Verification items for the finished model (mm, model axes). A direction names the side the tool comes from. Round coordinates to 2 decimals unless told otherwise and drop trailing zeros. Write each loop counter-clockwise with the first axis right and the second up, starting at its lowest first coordinate (ties: lowest second). Pieces come first, ordered by that corner, then holes.
from build123d import *

# Parameters (mm, degrees)
SKETCH_W        = 200
SKETCH_H        = 90
SKETCH_W_2      = 60
SKETCH_H_2      = 67
PAD_DEPTH       = 5
SKETCH001_W     = 200
SKETCH001_H     = 90
SKETCH001_W_2   = 124
SKETCH001_H_2   = 67
PAD001_DEPTH    = 5
SKETCH002_W     = 41
SKETCH002_H     = 9.5
POCKET_DEPTH    = 10.001
SKETCH003_R     = 1.5625
POCKET001_DEPTH = 10.001
FILLET_R        = 30
FILLET001_R     = 3
FILLET002_R     = 3
POCKET002_DEPTH = 2
FILLET003_R     = 1
FILLET004_R     = 1


with BuildPart() as part:
    # Sketch → Pad (new body)
    with BuildSketch(Plane.XY):
        with Locations((100, -45)):
            Rectangle(SKETCH_W, SKETCH_H)
        with Locations((70, -38.5)):
            Rectangle(SKETCH_W_2, SKETCH_H_2, mode=Mode.SUBTRACT)
        with BuildLine():
            ThreePointArc((158.0113, -7.9887), (155.0113, -4.9887), (152.0113, -7.9887))
            Line((152.0113, -7.9887), (152.0113, -17.9887))
            ThreePointArc((152.0113, -17.9887), (155.0113, -20.9887), (158.0113, -17.9887))
            Line((158.0113, -7.9887), (158.0113, -17.9887))
        make_face(mode=Mode.SUBTRACT)
        with BuildLine():
            ThreePointArc((151, -31.5), (131.5, -12), (112, -31.5))
            Line((112, -31.5), (112, -41.5))
            ThreePointArc((112, -41.5), (131.5, -61), (151, -41.5))
            Line((151, -31.5), (151, -41.5))
        make_face(mode=Mode.SUBTRACT)
        with BuildLine():
            ThreePointArc((158.0113, -55.0113), (155.0113, -52.0113), (152.0113, -55.0113))
            Line((152.0113, -55.0113), (152.0113, -65.0113))
            ThreePointArc((152.0113, -65.0113), (155.0113, -68.0113), (158.0113, -65.0113))
            Line((158.0113, -55.0113), (158.0113, -65.0113))
        make_face(mode=Mode.SUBTRACT)
        with BuildLine():
            ThreePointArc((110.9887, -55.0113), (107.9887, -52.0113), (104.9887, -55.0113))
            Line((104.9887, -55.0113), (104.9887, -65.0113))
            ThreePointArc((104.9887, -65.0113), (107.9887, -68.0113), (110.9887, -65.0113))
            Line((110.9887, -55.0113), (110.9887, -65.0113))
        make_face(mode=Mode.SUBTRACT)
        with BuildLine():
            ThreePointArc((110.9887, -7.9887), (107.9887, -4.9887), (104.9887, -7.9887))
            Line((104.9887, -7.9887), (104.9887, -17.9887))
            ThreePointArc((104.9887, -17.9887), (107.9887, -20.9887), (110.9887, -17.9887))
            Line((110.9887, -7.9887), (110.9887, -17.9887))
        make_face(mode=Mode.SUBTRACT)
    extrude(amount=PAD_DEPTH)

    # Sketch001 → Pad001 (join)
    with BuildSketch(Plane(origin=(0, 0, 0), x_dir=(1, 0, 0), z_dir=(0, 0, -1))):
        with Locations((100, 45)):
            Rectangle(SKETCH001_W, SKETCH001_H)
        with Locations((102, 38.5)):
            Rectangle(SKETCH001_W_2, SKETCH001_H_2, mode=Mode.SUBTRACT)
    extrude(amount=PAD001_DEPTH)

    # Sketch002 → Pocket (cut, through all)
    with BuildSketch(Plane.XY.offset(5)):
        with Locations((70, -76.75)):
            Rectangle(SKETCH002_W, SKETCH002_H)
    extrude(amount=-POCKET_DEPTH, mode=Mode.SUBTRACT)

    # Sketch003 → Pocket001 (cut, through all)
    with BuildSketch(Plane.XY.offset(5)):
        with Locations((25, -10)):
            Circle(SKETCH003_R)
        with Locations((15, -20)):
            Circle(SKETCH003_R)
        with Locations((15, -40)):
            Circle(SKETCH003_R)
        with Locations((25, -30)):
            Circle(SKETCH003_R)
        with Locations((175, -10)):
            Circle(SKETCH003_R)
        with Locations((185, -20)):
            Circle(SKETCH003_R)
        with Locations((185, -40)):
            Circle(SKETCH003_R)
        with Locations((175, -30)):
            Circle(SKETCH003_R)
    extrude(amount=-POCKET001_DEPTH, mode=Mode.SUBTRACT)

    # Fillet
    fillet_edges = [part.edges().sort_by_distance(p)[0] for p in [
        (0, -90, 2.5),
        (0, -90, -2.5),
        (200, -90, 2.5),
        (200, -90, -2.5),
    ]]
    fillet(fillet_edges, radius=FILLET_R)

    # Fillet001
    fillet001_edges = [part.edges().sort_by_distance(p)[0] for p in [
        (100, -5, 2.5),
        (40, -5, 2.5),
        (40, -5, -2.5),
        (49.5, -81.5, 0),
        (49.5, -72, 2.5),
        (49.5, -72, -2.5),
        (40, -72, 2.5),
        (40, -72, -2.5),
        (200, 0, 2.5),
        (200, 0, -2.5),
        (0, 0, 2.5),
        (0, 0, -2.5),
        (90.5, -81.5, 0),
        (90.5, -72, 2.5),
        (90.5, -72, -2.5),
    ]]
    fillet(fillet001_edges, radius=FILLET001_R)

    # Fillet002
    fillet002_edges = [part.edges().sort_by_distance(p)[0] for p in [
        (100, -72, 2.5),
    ]]
    fillet(fillet002_edges, radius=FILLET002_R)

    # Sketch004 (on Face1 of Fillet002) → Pocket002 (cut)
    with BuildSketch(Plane.XY.offset(5)):
        with BuildLine():
            ThreePointArc((161.5113, -7.9887), (155.0113, -1.4887), (148.5113, -7.9887))
            Line((148.5113, -7.9887), (148.5113, -17.9887))
            ThreePointArc((148.5113, -17.9887), (155.0113, -24.4887), (161.5113, -17.9887))
            Line((161.5113, -7.9887), (161.5113, -17.9887))
        make_face()
        with BuildLine():
            ThreePointArc((114.4887, -7.9887), (107.9887, -1.4887), (101.4887, -7.9887))
            Line((101.4887, -7.9887), (101.4887, -17.9887))
            ThreePointArc((101.4887, -17.9887), (107.9887, -24.4887), (114.4887, -17.9887))
            Line((114.4887, -7.9887), (114.4887, -17.9887))
        make_face()
        with BuildLine():
            ThreePointArc((114.4887, -55.0113), (107.9887, -48.5113), (101.4887, -55.0113))
            Line((101.4887, -55.0113), (101.4887, -65.0113))
            ThreePointArc((101.4887, -65.0113), (107.9887, -71.5113), (114.4887, -65.0113))
            Line((114.4887, -55.0113), (114.4887, -65.0113))
        make_face()
        with BuildLine():
            ThreePointArc((161.5113, -55.0113), (155.0113, -48.5113), (148.5113, -55.0113))
            Line((148.5113, -55.0113), (148.5113, -65.0113))
            ThreePointArc((148.5113, -65.0113), (155.0113, -71.5113), (161.5113, -65.0113))
            Line((161.5113, -55.0113), (161.5113, -65.0113))
        make_face()
    extrude(amount=-POCKET002_DEPTH, mode=Mode.SUBTRACT)

    # Fillet003
    fillet003_edges = [part.edges().sort_by_distance(p)[0] for p in [
        (200, -31.5, 5),
        (8.786797, -81.213203, 5),
        (100, -90, 5),
        (191.213203, -81.213203, 5),
        (0, -31.5, 5),
        (0.87868, -0.87868, 5),
        (100, 0, 5),
        (199.12132, -0.87868, 5),
    ]]
    fillet(fillet003_edges, radius=FILLET003_R)

    # Fillet004
    fillet004_edges = [part.edges().sort_by_distance(p)[0] for p in [
        (0, -31.5, -5),
        (8.786797, -81.213203, -5),
        (100, -90, -5),
        (191.213203, -81.213203, -5),
        (200, -31.5, -5),
        (0.87868, -0.87868, -5),
        (100, 0, -5),
        (199.12132, -0.87868, -5),
    ]]
    fillet(fillet004_edges, radius=FILLET004_R)


solid = part.part
Q1. Sectioned sample at A-A (x = 131.5). Enter the section's corners in (y, z), plus the area to 3 significant figures.
Recorded:
outline: (-90, -4) arc R1 ccw to (-89, -5) - (-72, -5) - (-72, 0) - (-61, 0) - (-61, 5) - (-89, 5) arc R1 ccw to (-90, 4) - close; (-12, 0) - (-5, 0) - (-5, -5) - (-1, -5) arc R1 ccw to (0, -4) - (0, 4) arc R1 ccw to (-1, 5) - (-12, 5) - close
area: 319 mm2
Q2. Sectioned sample at B-B (y = -36). Enter the section's corners in (x, z), plus the area to 3 significant figures.
Recorded:
outline: (0, -4) arc R1 ccw to (1, -5) - (40, -5) - (40, 5) - (1, 5) arc R1 ccw to (0, 4) - close; (100, 0) - (112, 0) - (112, 5) - (100, 5) - close; (151, 0) - (164, 0) - (164, -5) - (199, -5) arc R1 ccw to (200, -4) - (200, 4) arc R1 ccw to (199, 5) - (151, 5) - close
area: 884 mm2
Q3. Depth check by flat-ended pin: P1, Ø2, axis at y = -64.5, z = -3, coming from the -X side; P2, Ø3.5, axis at x = 185, y = -40, coming from the -Z side; P3, Ø1.5, axis at y = -62, z = 2, coming from the +X side. Enter the tip coordinate at first touch or a pass-through.
Recorded:
P1: stops at x = 0.2
P2: stops at z = -5
P3: stops at x = 199.97
Q4. Tool access check on faces 1 (the flat face through (151, -36, 2)), 2 (the cylindrical face through (154.868, -24.487, 4.014)), 3 (the flat face through (115, -53, 0)). Record the directions out of +Z, -Z, +X, -X, +Y, -Y that give a thin tool (end or side, any length) a straight path to the whole face; none if there is none.
Recorded:
face 1: +Z, -Z
face 2: +Z
face 3: -Z
Q5. Sectioned sample at C-C (z = 1.5). Give the number of separate pieces and of enclosed holes in the cut face, plus the area to 3 significant figures.
Recorded:
separate pieces: 1
enclosed holes: 14
area: 11,200 mm2
Q6. Material ranges on line 1 along X through (y, z) = (-8, 1.25); line 2 along X through (y, z) = (-37, 1.5); line 3 along Y through (x, z) = (132.5, -3.5), recorded low to high.
Recorded:
line 1: x = 0 to 40, 100 to 104.99, 110.99 to 152.01, 158.01 to 200
line 2: x = 0 to 40, 100 to 112, 151 to 200
line 3: y = -90 to -72, -5 to 0
Q7. Release check for a two-part mould opening along Y. For faces 4 (the flat face through (99, 0, 0)), 5 (the cylindrical face through (8.555, -80.979, 0.056)), 6 (the flat face through (112, -13, 3)), 7 (the flat face through (121, -64, 5)) record: released by +Y, released by -Y, zero draft, split by the parting line, or undercut.
Recorded:
face 4: released by +Y
face 5: released by -Y
face 6: undercut
face 7: zero draft
